```python
from build123d import *

# Parameters (mm, degrees)
F0_W     = 40
F0_H     = 20
F1_DEPTH = 6.35
F2_W     = 40
F2_H     = 6.35
F3_DEPTH = 44.15
F5_D     = 10.7188
F5_DEPTH = 12.7
F5_TIP   = 3.2202524016
F6_D     = 5.8
F6_DEPTH = 12.7
F6_TIP   = 1.7424957952


with BuildPart() as f1:
    # F0 (on Right) → F1 (new body)
    with BuildSketch(Plane.YZ):
        with Locations((20, 10)):
            Rectangle(F0_W, F0_H)
    extrude(amount=F1_DEPTH)

    # F2 (on face) → F3 (join)
    with BuildSketch(Plane(origin=(0, 0, 0), x_dir=(0, -1, 0), z_dir=(-1, 0, 0))):
        with Locations((-20, 3.175)):
            Rectangle(F2_W, F2_H)
    extrude(amount=F3_DEPTH)

    # F5
    with Locations(Plane.XY.offset(6.35)):
        with Locations((-18.75, 20)):
            Hole(F5_D / 2, depth=F5_DEPTH)
            with Locations((0, 0, -(F5_DEPTH + F5_TIP / 2))):  # 118° drill point
                Cone(0, F5_D / 2, F5_TIP, mode=Mode.SUBTRACT)

    # F6
    with Locations(Plane(origin=(0, 0, 0), x_dir=(0, 1, 0), z_dir=(-1, 0, 0))):
        with Locations((30, -14), (10, -14)):
            Hole(F6_D / 2, depth=F6_DEPTH)
            with Locations((0, 0, -(F6_DEPTH + F6_TIP / 2))):  # 118° drill point
                Cone(0, F6_D / 2, F6_TIP, mode=Mode.SUBTRACT)


solid = f1.part
```
For this review, take the finished solid that the model builds, in its own axes (mm). A direction names the side the tool comes from. Round coordinates to 2 decimals unless told otherwise and drop trailing zeros. Write each loop counter-clockwise with the first axis right and the second up, starting at its lowest first coordinate (ties: lowest second). Pieces come first, ordered by that corner, then holes.
1) Mouldability with a two-part tool opening along Y and no side actions: class faces 3 (the face through (3.219, 12.301, 15.765)), 4 (the face through (0, 20, 13)), 5 (the face through (-13, 40, 5)) as +Y half, -Y half, draft (parallel to the pull), parting line (faces both ways), or undercut.
Answer below:
face 3: undercut
face 4: draft
face 5: +Y half
2) Take a section at D-D on y = 10. Give the boundary of the cut face in (x, z).
Answer below:
outline: (-44.15, 0) - (6.35, 0) - (6.35, 11.1) - (0, 11.1) - (0, 6.35) - (-44.15, 6.35) - close; (0, 16.9) - (6.35, 16.9) - (6.35, 20) - (0, 20) - close
3) Machinability: for faces 1 (the face through (3, 20, 20)), 2 (the face through (-22, 25, 6.35)), which of the approach directions +Z, -Z, +X, -X, +Y, -Y give a long, thin tool a straight path to every point of the face, cutting with its end or side? Answer none if there is none.
Answer below:
face 1: +Z, +X, -X, +Y, -Y
face 2: +Z, -X, +Y, -Y
4) Take a section at C-C on x = -18.75. Give the boundary of the cut face in (y, z).
Answer below:
outline: (0, 0) - (14.64, 0) - (14.64, 6.35) - (0, 6.35) - close; (25.36, 0) - (40, 0) - (40, 6.35) - (25.36, 6.35) - close
5) Insertion check: pin 1 Ø12 at (x, y) = (-17.5, 5.5) entering from +Z; pin 2 Ø1 at (y, z) = (7.5, 15) entering from -X. Each pin has a flat end and moves straight along its axis. Give the tip position at first contact, or say it passes through.
Answer below:
pin 1: stops at z = 6.35
pin 2: stops at x = 0
6) Take a section at A-A on y = 20. Give the boundary of the cut face in (x, z).
Answer below:
outline: (-44.15, 0) - (-24.11, 0) - (-24.11, 6.35) - (-44.15, 6.35) - close; (-13.39, 0) - (6.35, 0) - (6.35, 20) - (0, 20) - (0, 6.35) - (-13.39, 6.35) - close
7) For line 1 along Y through (x, z) = (2.5, 14); line 2 along Z through (x, y) = (4, 10); line 3 along Y through (x, z) = (-18.5, 2.5), list the stretches that pass through material, from the lowest coordinate up.
Answer below:
line 1: y = 0 to 7.1, 12.9 to 27.1, 32.9 to 40
line 2: z = 0 to 11.1, 16.9 to 20
line 3: y = 0 to 14.65, 25.35 to 40
8) Take a section at B-B on z = 14. Give the boundary of the cut face in (x, y), then the cut area to 3 significant figures.
Answer below:
outline: (0, 0) - (6.35, 0) - (6.35, 7.1) - (0, 7.1) - close; (0, 12.9) - (6.35, 12.9) - (6.35, 27.1) - (0, 27.1) - close; (0, 32.9) - (6.35, 32.9) - (6.35, 40) - (0, 40) - close
area: 180 mm2
